Check sheet for the modelled part. Datum: model origin and axes. Units: mm. Face numbers are marked on the shaded views. A direction names the side the tool comes from. Give positions to 0.01 mm unless a question says otherwise; leave off trailing zeros. Write each loop counter-clockwise with the first axis right and the second up, starting at its lowest first coordinate (ties: lowest second). Pieces come first, ordered by that corner, then holes. Notation, with made-up numbers: (64.5, 63) -> (93.5, 63) arc R20 cw to (93.5, 74) -> close; hole circle Ø8 at (69.5, 84.25). An arc over 180 degrees is marked (long way). Answer as a JSON object with one key per item and string values.
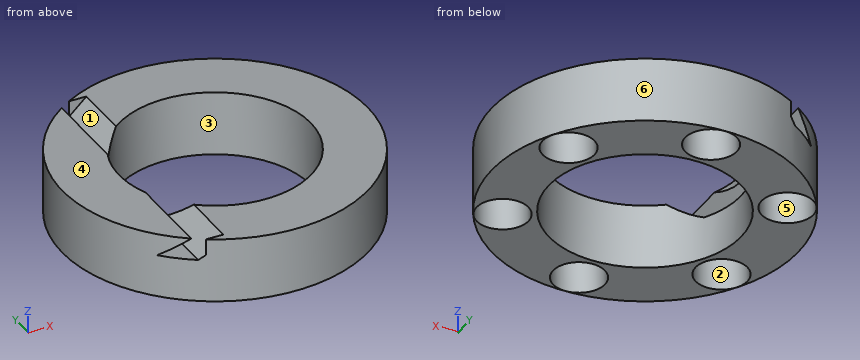
Autodesk Fusion 360 part; units mm, degrees
sketch "Sketch1" plane through (0, 0, 0) normal (0, 0, 1) x (1, 0, 0)
  circle A0 centre (0, 0) radius 22.225
  circle A1 centre (0, 0) radius 35.425
  circle A2 centre (0, 29.3625) radius 6
  circle A3 centre (-25.4287, 14.6813) radius 6
  circle A4 centre (-25.4287, -14.6812) radius 6
  circle A5 centre (0, -29.3625) radius 6
  circle A6 centre (25.4287, -14.6813) radius 6
  circle A7 centre (25.4287, 14.6812) radius 6
  dimension "d1" = 44.45
  dimension "d2" = 70.85
  dimension "d3" = 12
  dimension "d4" = 29.3625
  dimension "d6" = 360
extrude "Extrude1" add sketch "Sketch1" along normal blind 15 contours A1 | A2 | A3 | A4 | A5 | A6 | A7 makes body 1
extrude "Extrude2" cut sketch "Sketch1" along normal blind 9 contours A2 | A3 | A4 | A5 | A6 | A7 bodies 1
sketch "Sketch2" plane through (0, 0, 0) normal (0, 1, 0) x (1, 0, 0)
  line L0 (-15.955, -19.2911) -> (-26, -9.924)
  line L1 (-26, -9.924) -> (-19.4017, -9.924)
  line L2 (-19.4017, -9.924) -> (-12.886, -16)
  line L3 (-12.886, -16) -> (-15.955, -19.2911)
  line L4 (0, 0) -> (0, -30.1801) construction
  line L5 (-35.425, -15) -> (35.425, -15)
  dimension "d11" = 47
  dimension "d12" = 4.5
  dimension "d13" = 5.076
  dimension "d14" = 26
  dimension "d15" = 1
extrude "Extrude3" cut sketch "Sketch2" along normal mid plane 61 bodies 1
copy_body "Body->Comp1" bodies 1 removing the originals makes body 2 in component "Component"
sketch "Sketch3" plane through (0, 0, 0) normal (0, 1, 0) x (1, 0, 0)
  line L0 (0, -15) -> (50, -4)
  line L1 (50, -4) -> (50, -15)
  line L2 (0, -15) -> (50, -15)
  line L3 (-18.0189, -15) -> (35.425, -15)
  dimension "d19" = 50
  dimension "d25" = 11
component "Component" placed x (1, 0, 0) y (0, 1, 0) z (0, 0, 1) at (0, 0, 0)
1. Sectioned sample at C-C, the plane z = 4.25. State how many separate pieces and enclosed holes the cut face has, plus the area to 3 significant figures.
Determined:
{"separate pieces": "1", "enclosed holes": "7", "area": "1,710 mm^2"}
2. Go/stop test with flat-tipped pins: P1, Ø6, axis at y = 20, z = 9.5, coming from the -X side; P2, Ø3.5, axis at x = -23.5, y = 14, coming from the -Z side; P3, Ø1, axis at x = 18.5, z = 7, coming from the -Y side. Record where each tip stops, or that it passes through.
Determined:
{"P1": "x = -31.08", "P2": "z = 9", "P3": "y = -30.51"}
3. Sectioned sample at D-D, the plane y = -12.5. Enter the section's corners in (x, z).
Determined:
{"outline": "(-33.15, 0) -> (-31.02, 0) -> (-31.02, 9) -> (-19.84, 9) -> (-19.84, 0) -> (-18.38, 0) -> (-18.38, 10.88) -> (-19.4, 9.92) -> (-26, 9.92) -> (-20.56, 15) -> (-33.15, 15) -> close; (18.38, 0) -> (19.84, 0) -> (19.84, 9) -> (31.02, 9) -> (31.02, 0) -> (33.15, 0) -> (33.15, 15) -> (18.38, 15) -> close"}
4. Access from +Z, -Z, +X, -X, +Y, -Y to the whole of each face (thin tool, end or side, straight path). Record for the marked faces 1, 2 and 3.
Determined:
{"face 1": "+Z", "face 2": "-Z", "face 3": "+Z, -Z"}
5. Scan lines: L1, parallel to Y at x = 24.5, z = 6.75; L2, parallel to X at y = 20, z = 12.5; L3, parallel to X at y = -29, z = 2. Record each from-to range of solid material in increasing order. Write a range as [from, to].
Determined:
{"L1": "[-25.59, -20.61], [-8.75, 8.75], [20.61, 25.59]", "L2": "[-29.24, -23.24], [-16.64, -9.69], [9.69, 29.24]", "L3": "[-20.35, -5.99], [5.99, 20.35]"}
6. Mould release check, pull along X, two halves, no side actions. Record for the marked faces 4, 5 and 6: released by +X, released by -X, zero draft, split by the parting line, or undercut.
Determined:
{"face 4": "zero draft", "face 5": "undercut", "face 6": "split by the parting line"}
7. Sectioned sample at B-B, the plane y = 0. Enter the section's corners in (x, z) (3 decimals), plus the area to 3 significant figures.
Determined:
{"outline": "(-35.425, 0) -> (-22.225, 0) -> (-22.225, 9.924) -> (-26, 9.924) -> (-22.225, 13.444) -> (-22.225, 15) -> (-35.425, 15) -> close; (22.225, 0) -> (35.425, 0) -> (35.425, 15) -> (22.225, 15) -> close", "area": "389 mm^2"}
